Could you check a few things on this model? Use its own coordinates, in mm. Coordinates: 2 decimals unless noted, no trailing zeros. Write each loop counter-clockwise with the first axis right and the second up, starting at its lowest first coordinate (ties: lowest second). Pieces come first, ordered by that corner, then holes.
Item 1: If I drill on probe 1 along Z at (x, y) = (0, -18.5); probe 2 along Y at (x, z) = (0, 378); probe 3 along X at (y, z) = (1, 109), over which ranges is the centre line in solid material (lowest first)?
Item 2: I want a section at B-B on x = 10. Please give me the cut outline in (y, z), then the cut area to 3 significant figures.
Item 3: For P1, Ø4, axis at x = 13, z = 261.5, coming from the +Y side; P2, Ø1.5, axis at x = -9, z = 462.5, coming from the +Y side; P3, Ø5, axis at x = 7, z = 466, coming from the -Y side, each with a flat end and sliding along its axis, tell me the tip position at first contact or that it passes through.
Item 4: I want a section at A-A on y = 0. Please give me the cut outline in (x, z), then the cut area to 3 significant figures.
Item 5: I want a section at C-C on z = 217. Please give me the cut outline in (x, y).
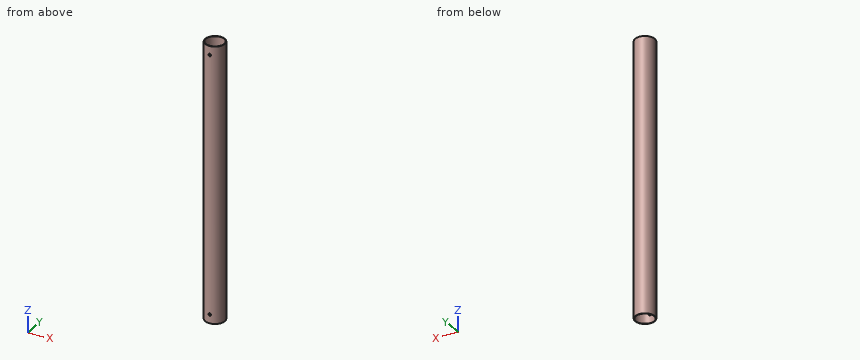
from build123d import *

# Parameters (mm, degrees)
ESQUISSE1_R             = 19
ESQUISSE1_R_2           = 18
BOSS_EXTRU_1_DEPTH      = 530
ESQUISSE2_R             = 2.5
ENL_V_MAT_EXTRU_1_DEPTH = 531.680694957
ESQUISSE4_R             = 2.5
ENL_V_MAT_EXTRU_2_DEPTH = 531.680695064


with BuildPart() as part:
    # Esquisse1 → Boss.-Extru.1 (new body)
    with BuildSketch(Plane.XY):
        Circle(ESQUISSE1_R)
        Circle(ESQUISSE1_R_2, mode=Mode.SUBTRACT)
    extrude(amount=BOSS_EXTRU_1_DEPTH)

    # Esquisse2 → Enlèv. mat.-Extru.1 (cut, through all)
    with BuildSketch(Plane(origin=(0, 0, 0), x_dir=(1, 0, 0), z_dir=(0, 1, 0))):
        with Locations(Location((0, -17, 0), (0, 0, 270))):
            Circle(ESQUISSE2_R)
    extrude(amount=-ENL_V_MAT_EXTRU_1_DEPTH, mode=Mode.SUBTRACT)

    # Esquisse4 → Enlèv. mat.-Extru.2 (cut, through all)
    with BuildSketch(Plane(origin=(0, 0, 0), x_dir=(1, 0, 0), z_dir=(0, 1, 0))):
        with Locations(Location((0, -513, 0), (0, 0, 270))):
            Circle(ESQUISSE4_R)
    extrude(amount=-ENL_V_MAT_EXTRU_2_DEPTH, mode=Mode.SUBTRACT)


solid = part.part
Response values:
1. probe 1: z = 0 to 14.5, 19.5 to 510.5, 515.5 to 530
1. probe 2: y = -19 to -18, 18 to 19
1. probe 3: x = -18.97 to -17.97, 17.97 to 18.97
2. outline: (-16.16, 0) - (-14.97, 0) - (-14.97, 530) - (-16.16, 530) - close; (14.97, 0) - (16.16, 0) - (16.16, 530) - (14.97, 530) - close
2. area: 1,260 mm2
3. P1: stops at y = 15.49
3. P2: stops at y = 17.12
3. P3: stops at y = -18.46
4. outline: (-19, 0) - (-18, 0) - (-18, 530) - (-19, 530) - close; (18, 0) - (19, 0) - (19, 530) - (18, 530) - close
4. area: 1,060 mm2
5. outline: circle Ø38 at (0, 0); hole circle Ø36 at (0, 0)
